Job drawing, mm, ordinate dimensions from the low corner. One solid piece. A direction names the side the tool comes from. Give positions to 0.01 mm unless a question says otherwise; leave off trailing zeros. Write each loop counter-clockwise with the first axis right and the second up, starting at its lowest first coordinate (ties: lowest second). Pieces come first, ordered by that corner, then holes. Notation, with made-up numbers: M 85,-20.5 L 129,-20.5 A20 cw 129,8.5 Z; hole C -9.5,-39 d10. An arc over 180 degrees is marked long. Answer as CSV lines item,"result". Start each with the question number.
1) Wall check: line 1 along Z through (x, y) = (12.5, 14); line 2 along Z through (x, y) = (8.5, 1.75); line 3 along Y through (x, z) = (12, 38). Give the ranges that are in metal, low to high. Write a range as from..to.
2) Slice it at C-C, the plane x = 8.25. Give the cut face in (y, z).
3) Tool access for the marked faces 1 and 2: list every direction of +Z, -Z, +X, -X, +Y, -Y with a clear straight run to the whole face (end or side of a thin tool).
4) Slice it at B-B, the plane x = 12.5. Give the cut face in (y, z).
5) Slice it at A-A, the plane y = 12.5. Give the cut face in (x, z), plus the area to 3 significant figures.
6) Slice it at D-D, the plane z = 50.5. Give the cut face in (x, y).
7) Pin check, flat tips, straight feed: pin 1 Ø3 at (y, z) = (19.5, 72.5) entering from -X; pin 2 Ø10 at (x, z) = (17.5, 52.5) entering from -Y; pin 3 Ø10 at (y, z) = (7, 53) entering from +X; pin 4 Ø1 at (x, z) = (2.5, 94) entering from +Y. Stop position of each tip, or through.
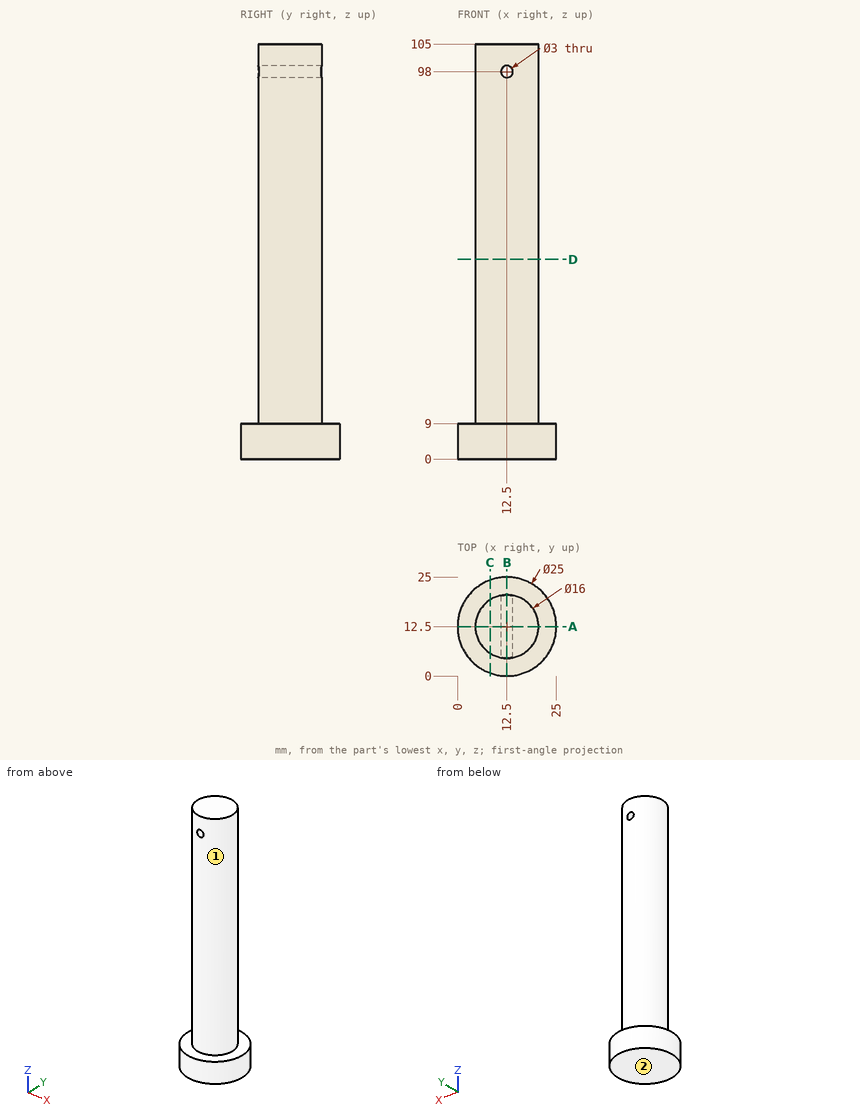
Found:
1,line 1,"0..96.5, 99.5..105"
1,line 2,"0..9"
1,line 3,"4.52..20.48"
2,outline,"M 0.74,0 L 24.26,0 L 24.26,9 L 19.28,9 L 19.28,105 L 5.72,105 L 5.72,9 L 0.74,9 Z"
3,face 1,"+Z"
3,face 2,"-Z, +X, -X, +Y, -Y"
4,outline,"M 0,0 L 25,0 L 25,9 L 20.5,9 L 20.5,96.5 L 4.5,96.5 L 4.5,9 L 0,9 Z; M 4.5,99.5 L 20.5,99.5 L 20.5,105 L 4.5,105 Z"
5,outline,"M 0,0 L 25,0 L 25,9 L 20.5,9 L 20.5,105 L 4.5,105 L 4.5,9 L 0,9 Z; hole C 12.5,98 d3"
5,area,"1,750 mm²"
6,outline,"C 12.5,12.5 d16"
7,pin 1,"x = 6.69"
7,pin 2,"y = 4.5"
7,pin 3,"x = 20.48"
7,pin 4,"through"
